from build123d import *

# Parameters (mm, degrees)
SKETCH_1_R               = 60
SKETCH_1_R_2             = 14.438127561
EXTRUDE_1_DEPTH          = 40
CHAMFER_1_SIZE           = 2
SKETCH_5_R               = 25.161734689
EXTRUDE_2_DEPTH          = 40
CUT_EXTRUDE_1_DEPTH      = 776.044855896
CUT_EXTRUDE_1_DEPTH_BACK = 776.044855896
CHAMFER_2_SIZE           = 1.361088561
CHAMFER_2_SIZE_2         = 1


with BuildPart() as part:
    # 草图1 → 凸台-拉伸1 (new body)
    with BuildSketch(Plane.XY.offset(70.26)):
        with Locations((-297.670899951, 626.415366791)):
            Circle(SKETCH_1_R)
        with Locations((-297.670899951, 626.415366791)):
            Circle(SKETCH_1_R_2, mode=Mode.SUBTRACT)
    extrude(amount=-EXTRUDE_1_DEPTH)

    # 草图4 → 切除-旋转1 (revolve, cut)
    with BuildSketch(Plane(origin=(0, 626.415366791, 0), x_dir=(1, 0, 0), z_dir=(0, 1, 0))):
        with BuildLine():
            Line((-244.095308656, -48.103310059), (-244.095308655, -52.416689982))
            ThreePointArc((-244.095308655, -52.416689982), (-242.284199059, -57.48597347), (-237.670899813, -60.259999987))
            Line((-237.670899813, -60.259999987), (-237.670899811, -40.260000013))
            ThreePointArc((-237.670899811, -40.260000013), (-242.284199071, -43.034026546), (-244.095308656, -48.103310059))
        make_face()
    revolve(axis=Axis((-299.491656028, 626.415366791, 70.26), (0, 0, -1)), mode=Mode.SUBTRACT)

    # 倒角1
    chamfer_1_edges = [part.edges().sort_by_distance(p)[0] for p in [
        (-357.670899951, 626.415366791, 70.26),
        (-357.670899951, 626.415366791, 30.26),
    ]]
    chamfer(chamfer_1_edges, length=CHAMFER_1_SIZE)

    # 草图5 → 凸台-拉伸2 (add)
    with BuildSketch(Plane.XY.offset(70.26)):
        with Locations((-297.670899951, 626.415366791)):
            Circle(SKETCH_5_R)
    extrude(amount=-EXTRUDE_2_DEPTH)

    # 草图6 → 切除-拉伸1 (cut, two sides: drawn at the far end of the back side and taken through both)
    with BuildSketch(Plane(origin=(0, 0, 30.26), x_dir=(-1, 0, 0), z_dir=(0, 0, -1)).offset(-CUT_EXTRUDE_1_DEPTH_BACK)):
        with BuildLine():
            ThreePointArc((302.170899951, 644.874781733), (297.670899951, 645.415366791), (293.170899951, 644.874781733))
            Line((293.170899951, 644.874781733), (293.170899951, 626.415366791))
            Line((293.170899951, 626.415366791), (302.170899951, 626.415366791))
            Line((302.170899951, 626.415366791), (302.170899951, 644.874781733))
        make_face()
        with BuildLine():
            Line((293.170899951, 626.415366791), (293.170899951, 644.874781733))
            ThreePointArc((293.170899951, 644.874781733), (285.934205356, 611.473813993), (316.670899951, 626.415366791))
            ThreePointArc((316.670899951, 626.415366791), (312.612452748, 638.152061385), (302.170899951, 644.874781733))
            Line((302.170899951, 644.874781733), (302.170899951, 626.415366791))
            Line((302.170899951, 626.415366791), (293.170899951, 626.415366791))
        make_face()
        with BuildLine():
            Line((302.170899951, 648.095366791), (293.170899951, 648.095366791))
            Line((293.170899951, 648.095366791), (293.170899951, 644.874781733))
            ThreePointArc((293.170899951, 644.874781733), (297.670899951, 645.415366791), (302.170899951, 644.874781733))
            Line((302.170899951, 644.874781733), (302.170899951, 648.095366791))
        make_face()
    extrude(amount=CUT_EXTRUDE_1_DEPTH + CUT_EXTRUDE_1_DEPTH_BACK, mode=Mode.SUBTRACT)

    # 倒角2
    # the kernel refuses this chamfer: 1.361088561, 1 mm, written as the material it takes off along each edge
    with BuildSketch(Plane(origin=(-302.170899951, 644.874781733, 26.740268541), x_dir=(0, 1, 0), z_dir=(0, 0, 1))) as chamfer_2_piece_1:
        with BuildLine():
            Line((CHAMFER_2_SIZE, 0), (-0.270460462, 0.991988248))
            ThreePointArc((-0.270460462, 0.991988248), (-0.133734106, 0.516913582), (0, 0))
            Line((0, 0), (CHAMFER_2_SIZE, 0))
        make_face()
    extrude(amount=47.039462917, mode=Mode.SUBTRACT)
    with BuildSketch(Plane(origin=(-293.170899951, 644.874781733, 26.506479775), x_dir=(0, 1, 0), z_dir=(0, 0, 1))) as chamfer_2_piece_2:
        with BuildLine():
            Line((CHAMFER_2_SIZE_2, 0), (-0.398045781, -1.398045781))
            ThreePointArc((-0.398045781, -1.398045781), (-0.192184694, -0.725734308), (0, 0))
            Line((0, 0), (CHAMFER_2_SIZE_2, 0))
        make_face()
    extrude(amount=47.507040451, mode=Mode.SUBTRACT)
    # the kernel refuses this chamfer: 1.361088561, 1 mm, written as the material it takes off along each edge
    with BuildSketch(Plane(origin=(-297.670899951, 626.415366791, 30.26), x_dir=(0.17889175862136222, 0.9838687609114116, 0), z_dir=(-0.9838687609114116, 0.17889175862136222, 0))) as chamfer_2_2_piece_1:
        Polygon((19, -CHAMFER_2_SIZE_2), (19 + CHAMFER_2_SIZE_2, 0), (19, 0), align=None)
    revolve(axis=Axis((-297.670899951, 626.415366791, 30.26), (0, 0, -1)), revolution_arc=259.694785461, mode=Mode.SUBTRACT)
    with BuildSketch(Plane(origin=(-297.670899951, 626.415366791, 70.26), x_dir=(0.17889175862137457, 0.9838687609114093, 0), z_dir=(-0.9838687609114093, 0.17889175862137457, 0))) as chamfer_2_2_piece_2:
        Polygon((19 + CHAMFER_2_SIZE_2, 0), (19, CHAMFER_2_SIZE_2), (19, 0), align=None)
    revolve(axis=Axis((-297.670899951, 626.415366791, 70.26), (0, 0, -1)), revolution_arc=259.694785461, mode=Mode.SUBTRACT)
    with BuildSketch(Plane(origin=(-297.670899951, 626.415366791, 70.26), x_dir=(-1, 0, 0), z_dir=(0, -1, 0))) as chamfer_2_2_piece_3:
        Polygon((19 + CHAMFER_2_SIZE_2, 0), (19, CHAMFER_2_SIZE_2), (19, 0), align=None)
    revolve(axis=Axis((-297.670899951, 626.415366791, 70.26), (0, 0, -1)), revolution_arc=80.955933819, mode=Mode.SUBTRACT)
    with BuildSketch(Plane(origin=(-297.670899951, 626.415366791, 30.26), x_dir=(-1, 0, 0), z_dir=(0, -1, 0))) as chamfer_2_2_piece_4:
        Polygon((19, -CHAMFER_2_SIZE_2), (19 + CHAMFER_2_SIZE_2, 0), (19, 0), align=None)
    revolve(axis=Axis((-297.670899951, 626.415366791, 30.26), (0, 0, -1)), revolution_arc=80.955933819, mode=Mode.SUBTRACT)


solid = part.part
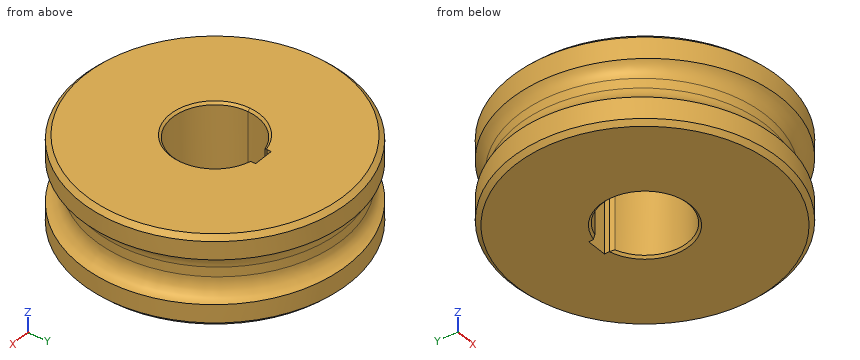
For this review, take the finished solid that the model builds, in its own axes (mm). Round coordinates to 2 decimals unless told otherwise and drop trailing zeros. Order: outer loops, then holes, each group sorted by start corner. A loop starts at its lowest first (then second) coordinate and runs counter-clockwise, first axis right, second up. Notation, with made-up numbers: (6, 26.25) -> (38, 26.25) arc R15 ccw to (38, 33.25) -> close; hole circle Ø4 at (49.25, 41.5). An arc over 180 degrees is marked (long way). Write item = value, one per line. Start each with the question number.
1) Take a section at A-A on z = 34. State the section outline as (x, y) points, plus the area to 3 significant figures.
2) Take a section at B-B on z = 46. State the section outline as (x, y) points.
3) Insertion check: pin 1 (1.5 mm diameter, centred on y = 616.5, z = 45.5, fed in from +X); pin 2 (1 mm diameter, centred on x = -315, z = 53.5, fed in from +Y); pin 3 (12 mm diameter, centred on x = -314, z = 62.5, fed in from +Y); pin 4 (1 mm diameter, centred on x = -343.5, y = 584.5, fed in from +Z). Each pin has a flat end and moves straight along its axis. Give the tip position at first contact, or say it passes through.
4) To check wall thickness, follow line 1 (X direction, y = 626.5, z = 62); line 2 (Y direction, x = -281.5, z = 49); line 3 (X direction, y = 614.5, z = 57.5). State the ranges of each line that lie inside material, in increasing order. Write a range as from..to.
Verdict:
q1.outline = circle Ø120 at (-297.67, 626.42); hole (-303.16, 644.6) arc R19 ccw (long way) to (-291.77, 644.48) -> (-293.17, 645.87) -> (-293.17, 648.1) -> (-302.17, 648.1) -> (-302.17, 646.24) -> close
q1.area = 10,100 mm2
q2.outline = circle Ø111.36 at (-299.49, 626.42); hole (-303.16, 644.6) arc R19 ccw (long way) to (-291.77, 644.48) -> (-293.17, 645.87) -> (-293.17, 648.1) -> (-302.17, 648.1) -> (-302.17, 646.24) -> close
q3.pin_1 = -244.22
q3.pin_2 = 679.84
q3.pin_3 = 685.52
q3.pin_4 = through
q4.line_1 = -357.67..-316.67, -278.67..-237.67
q4.line_2 = 574.02..616.44, 636.39..678.81
q4.line_3 = -355.46..-312.47, -282.87..-243.53
